```python
from build123d import *

# Parameters (mm, degrees)
SKETCH1_R           = 2.413
REVOLVE1_ANGLE      = 180
SKETCH2_R           = 2.413
BOSS_EXTRUDE1_DEPTH = 241.3
SKETCH3_R           = 2.413
BOSS_EXTRUDE2_DEPTH = 241.3


with BuildPart() as part:
    # Sketch1 → Revolve1 (revolve)
    with BuildSketch(Plane.XZ.offset(-215.9)):
        with Locations((152.4, 0)):
            Circle(SKETCH1_R)
    revolve(axis=Axis((76.2, 215.9, 2.413), (0, 0, 1)), revolution_arc=REVOLVE1_ANGLE)

    # Sketch2 → Boss-Extrude1 (add)
    with BuildSketch(Plane.XZ.offset(-215.9)):
        with Locations((152.4, 0)):
            Circle(SKETCH2_R)
    extrude(amount=BOSS_EXTRUDE1_DEPTH)

    # Sketch3 → Boss-Extrude2 (add)
    with BuildSketch(Plane.XZ.offset(-215.9)):
        Circle(SKETCH3_R)
    extrude(amount=BOSS_EXTRUDE2_DEPTH)


solid = part.part
```
Check sheet for the modelled part. Datum: model origin and axes. Units: mm. Round coordinates to 2 decimals unless told otherwise and drop trailing zeros. Order: outer loops, then holes, each group sorted by start corner. A loop starts at its lowest first (then second) coordinate and runs counter-clockwise, first axis right, second up. Notation, with made-up numbers: (-13.75, 62.25) -> (0.25, 62.25) arc R19 cw to (0.25, 79.25) -> close; hole circle Ø8 at (76.25, -14). An arc over 180 degrees is marked (long way). Use CSV: the item, a comma, the result in double quotes.
(1) Material ranges on line 1 along X through (y, z) = (153, -0.55); line 2 along X through (y, z) = (115, -0.2); line 3 along Y through (x, z) = (49, 1.25), recorded low to high. Write a range as from..to.
Worked out:
line 1,"-2.35..2.35, 150.05..154.75"
line 2,"-2.4..2.4, 150..154.8"
line 3,"284.87..289.29"
(2) Cross-section at A-A (z = 0). Record the boundary of the cut face in (x, y).
Worked out:
outline,"(-2.41, -25.4) -> (2.41, -25.4) -> (2.41, 215.9) arc R73.79 cw to (149.99, 215.9) -> (149.99, -25.4) -> (154.81, -25.4) -> (154.81, 215.9) arc R78.61 ccw to (-2.41, 215.9) -> close"
(3) Cross-section at B-B (y = 139). Record the boundary of the cut face in (x, z).
Worked out:
outline,"circle Ø4.83 at (0, 0); circle Ø4.83 at (152.4, 0)"
(4) Depth check by flat-ended pin: pin 1 (1 mm diameter, centred on x = 69, z = 0.5, fed in from -Y); pin 2 (2 mm diameter, centred on x = 40, z = 2, fed in from -Y); pin 3 (1.5 mm diameter, centred on x = 32, z = -0.5, fed in from +Y). Enter the tip coordinate at first touch or a pass-through.
Worked out:
pin 1,"y = 289.3"
pin 2,"y = 280.22"
pin 3,"y = 281.37"
